Input: part model. Units: mm. Frame: model coordinates. Coordinates: 2 decimals unless noted, no trailing zeros. Write each loop counter-clockwise with the first axis right and the second up, starting at its lowest first coordinate (ties: lowest second). Pieces come first, ordered by that corner, then holes. Notation, with made-up numbers: (22.5, -2.5) - (43.5, -2.5) arc R30 ccw to (43.5, 19.5) - close; hole circle Ø3 at (36, 70.25). An arc over 180 degrees is marked (long way). Put each result on its own line as item: value. Start each with the question number.
1. Line query: line 1 (X direction, y = 59, z = -3); line 2 (X direction, y = 62, z = -2); line 3 (X direction, y = 95, z = 2.75). Output: solid intervals per line, ascending.
2. Pull-direction query (X, two-part tool) for faces 1 (the cylindrical face through (-2.493, 55.694, -0.098)), 2 (the cylindrical face through (47.28, 43.4, 6.93)), 3 (the flat face through (-1, 39, 7.5)); classes: released by +X, released by -X, zero draft, split by the parting line, or undercut.
3. Cut plane B-B, the plane z = -2.25. Return loops of the section in (x, y), and give its area (3 significant figures).
4. Pin query (flat end, axial travel): pin 1 (6 mm diameter, centred on x = 37.5, z = 1.5, fed in from +Y); pin 2 (8 mm diameter, centred on y = 11.5, z = 5, fed in from -X); pin 3 (4 mm diameter, centred on x = 41.5, z = 2, fed in from +Y). Return the tip coordinate at first contact, or that it passes through.
5. Cut plane A-A, the plane x = 0. Return loops of the section in (y, z).
from build123d import *

# Parameters (mm, degrees)
SKETCH1_R           = 11.5
BOSS_EXTRUDE1_DEPTH = 7.5
FILLET1_R           = 2
CHAMFER1_SIZE       = 0.5


with BuildPart() as part:
    # Sketch1 → Boss-Extrude1 (new, symmetric)
    with BuildSketch(Plane.XY):
        with BuildLine():
            Line((-70, 0), (70, 0))
            Line((70, 0), (25, 88.582893039))
            ThreePointArc((25, 88.582893039), (0, 100), (-25, 88.582893039))
            Line((-25, 88.582893039), (-70, 0))
        make_face()
        with Locations((0, 66.920239342)):
            Circle(SKETCH1_R, mode=Mode.SUBTRACT)
    extrude(amount=BOSS_EXTRUDE1_DEPTH, both=True)

    # Fillet1
    # the kernel refuses this fillet: 2 mm, written as the material it takes off along each edge
    with BuildSketch(Plane(origin=(72.264547882, -4.457782284, 7.5), x_dir=(0, 0, -1), z_dir=(-0.45290957632946743, 0.8915564568040896, 0)), Plane(origin=(-22.735452118, 93.040675323, 7.5), x_dir=(0, 0, -1), z_dir=(-0.45290957632946743, -0.8915564568040896, 0))) as fillet1_piece_1:
        with BuildLine():
            CenterArc((FILLET1_R, FILLET1_R), FILLET1_R, 180, 90)
            Line((0, FILLET1_R), (0, 0))
            Line((0, 0), (FILLET1_R, 0))
        make_face()
    extrude(amount=109.357581186, mode=Mode.SUBTRACT)
    with BuildSketch(Plane(origin=(0, 66.920239342, 7.5), x_dir=(0.8457767754384001, 0.5335369210551618, 0), z_dir=(0.5335369210551618, -0.8457767754384001, 0))) as fillet1_piece_2:
        with BuildLine():
            CenterArc((33.079760658 - FILLET1_R, -FILLET1_R), FILLET1_R, 0, 90)
            Line((33.079760658 - FILLET1_R, 0), (33.079760658, 0))
            Line((33.079760658, 0), (33.079760658, -FILLET1_R))
        make_face()
    revolve(axis=Axis((0, 66.920239342, 7.5), (0, 0, 1)), revolution_arc=115.510513381, mode=Mode.SUBTRACT)
    with BuildSketch(Plane(origin=(0, 66.920239342, -7.5), x_dir=(0.8457767754384001, 0.5335369210551618, 0), z_dir=(0.5335369210551618, -0.8457767754384001, 0))) as fillet1_piece_3:
        with BuildLine():
            CenterArc((33.079760658 - FILLET1_R, FILLET1_R), FILLET1_R, 270, 90)
            Line((33.079760658 - FILLET1_R, 0), (33.079760658, 0))
            Line((33.079760658, 0), (33.079760658, FILLET1_R))
        make_face()
    revolve(axis=Axis((0, 66.920239342, -7.5), (0, 0, 1)), revolution_arc=115.510513381, mode=Mode.SUBTRACT)
    with BuildSketch(Plane(origin=(72.264547882, -4.457782284, -7.5), x_dir=(0, 0, 1), z_dir=(-0.45290957632946743, 0.8915564568040896, 0)), Plane(origin=(-22.735452118, 93.040675323, -7.5), x_dir=(0, 0, 1), z_dir=(-0.45290957632946743, -0.8915564568040896, 0))) as fillet1_piece_4:
        with BuildLine():
            CenterArc((FILLET1_R, -FILLET1_R), FILLET1_R, 90, 90)
            Line((0, -FILLET1_R), (0, 0))
            Line((0, 0), (FILLET1_R, 0))
        make_face()
    extrude(amount=109.357581186, mode=Mode.SUBTRACT)

    # Chamfer1
    chamfer1_edges = [part.edges().sort_by_distance(p)[0] for p in [
        (-11.5, 66.920239342, -7.5),
        (-11.5, 66.920239342, 7.5),
    ]]
    chamfer(chamfer1_edges, length=CHAMFER1_SIZE)


solid = part.part
Report:
1. line 1: x = -40.03 to -8.34, 8.34 to 40.03
1. line 2: x = -38.5 to -10.39, 10.39 to 38.5
1. line 3: x = -17.49 to 17.49
2. face 1: undercut
2. face 2: released by +X
2. face 3: zero draft
3. outline: (-70, 0) - (70, 0) - (25, 88.58) arc R33.08 ccw to (-25, 88.58) - close; hole circle Ø23 at (0, 66.92)
3. area: 8,400 mm^2
4. pin 1: stops at y = 69.88
4. pin 2: stops at x = -66.19
4. pin 3: stops at y = 60.04
5. outline: (0, -7.5) - (54.92, -7.5) - (55.42, -7) - (55.42, 7) - (54.92, 7.5) - (0, 7.5) - close; (78.42, -7) - (78.92, -7.5) - (98, -7.5) arc R2 ccw to (100, -5.5) - (100, 5.5) arc R2 ccw to (98, 7.5) - (78.92, 7.5) - (78.42, 7) - close
